Check sheet for the modelled part. Datum: model origin and axes. Units: mm. A direction names the side the tool comes from. Coordinates: 2 decimals unless noted, no trailing zeros. Write each loop counter-clockwise with the first axis right and the second up, starting at its lowest first coordinate (ties: lowest second). Pieces come first, ordered by that corner, then holes. Notation, with made-up numbers: (-29.5, 58) -> (7.5, 58) arc R31 ccw to (7.5, 93) -> close; hole circle Ø2 at (15, 62.5). An arc over 180 degrees is marked (long way). One line per item, written item: value. Start each with the question number.
1) Sectioned sample at B-B on z = 23.5. Enter the section's corners in (x, y).
2) Sectioned sample at C-C on x = -4. Enter the section's corners in (y, z).
3) Set-up check for faces 1 (the flat face through (-20, 0, 20)), 2 (the cylindrical face through (-53.987, 14.298, 5.07)), 3 (the flat face through (31, 5, 10)): record each of +Z, -Z, +X, -X, +Y, -Y from which the full face is reachable in a straight line by a thin tool's end or side.
4) Sectioned sample at A-A on y = 7. Give the number of separate pieces and of enclosed holes in the cut face, plus the area to 3 significant figures.
5) Scan lines: line 1 along X through (y, z) = (0, 4); line 2 along Y through (x, z) = (40, 4); line 3 along Z through (x, y) = (0, 4.5). Record each from-to range of solid material in increasing order. Write a range as [from, to].
6) Gauge pin test, flat ends, axial feed: P1, Ø2, axis at y = -16, z = 18, coming from the +X side; P2, Ø10, axis at y = -11, z = 33, coming from the -X side; P3, Ø18, axis at x = 40, y = 0, coming from the +Z side; P4, Ø5, axis at y = -6.5, z = 6, coming from the -X side. Record the tip position at first contact, or that the pin passes through.
7) Draft check along Y on faces 4 (the flat face through (-27, 0, 10)), 5 (the cylindrical face through (53.987, -14.298, 5.07)), 6 (the cylindrical face through (49.76, -2.17, 5.07)). Enter one of: +Y half, -Y half, draft (parallel to the pull), parting line (faces both ways), or undercut.
Autodesk Fusion 360 part; units mm, degrees
sketch "Sketch1" plane through (0, 0, 0) normal (0, 0, 1) x (1, 0, 0)
  line L0 (40, 20) -> (-40, 20)
  line L1 (-40, 20) -> (-40, -20)
  line L2 (-40, -20) -> (40, -20)
  line L3 (40, -20) -> (40, 20)
  line L4 (40, 20) -> (-40, -20) construction
  line L5 (-40, 20) -> (40, -20) construction
  line L6 (-40, -20) -> (-20, -20) construction
  line L7 (-40, -20) -> (-20, -20) construction
  line L8 (40, -20) -> (20, -20) construction
  line L9 (-20, -20) -> (-20, 20)
  line L10 (20, -20) -> (20, 20)
  line L11 (-40, -20) -> (-60, -20)
  line L12 (-40, 20) -> (-60, 20)
  line L13 (-60, 20) -> (-60, -20)
  line L14 (40, 20) -> (60, 20)
  line L15 (60, 20) -> (60, -20)
  line L16 (60, -20) -> (40, -20)
  line L17 (-40, 0) -> (-40, 20) construction
  line L18 (40, 20) -> (40, 0) construction
  dimension "d1" = 80
  dimension "d2" = 40
  dimension "d3" = 20
  dimension "d4" = 20
  dimension "d5" = 20
extrude "Extrude2" add sketch "Sketch1" along normal blind 50 contours L0 L2 L9 L10 makes body 1
extrude "Extrude1" add sketch "Sketch1" along normal blind 10 separate body contours L0 L2 L3 L10 | L3 L14 L15 L16 | L0 L1 L2 L9 | L1 L11 L12 L13 makes body 2 at (-33.3333, -6.6667, 0) makes body 3 at (46.6667, -6.6667, 0)
fillet "Fillet1" radius 20 4 edges at (-60, -20, 5) (-60, 20, 5) (60, -20, 5) (60, 20, 5) on bodies 2 3
hole "Hole1" at (-40, 0, 0) direction (0, 0, 1) diameter 20 depth 10 tip angle 118 bodies 2
hole "Hole2" at (40, 0, 0) direction (0, 0, 1) diameter 20 depth 10 tip angle 118 bodies 3
fillet "Fillet2" radius 20 2 edges at (-20, 0, 50) (20, 0, 50) on bodies 1
sketch "Sketch2" plane through (0, -20, 0) normal (0, -1, 0) x (1, 0, 0)
  arc A0 (20, 30) -> (-20, 30) centre (0, 30) ccw
  line L0 (-20, 30) -> (-20, 0)
  line L1 (-20, 0) -> (20, 0)
  line L2 (20, 0) -> (20, 30)
  line L3 (-20, 30) -> (20, 30) construction
hole "Hole3" at (0, -20, 30) direction (0, 1, 0) diameter 20 depth 40 tip angle 118 bodies 1
combine "Combine1" operation add target body 2 tool bodies 3 1
Answers:
1. outline: (-20, -20) -> (-7.6, -20) -> (-7.6, 20) -> (-20, 20) -> close; (7.6, -20) -> (20, -20) -> (20, 20) -> (7.6, 20) -> close
2. outline: (-20, 0) -> (20, 0) -> (20, 20.83) -> (-20, 20.83) -> close; (-20, 39.17) -> (20, 39.17) -> (20, 49.6) -> (-20, 49.6) -> close
3. face 1: +Z, -X, +Y, -Y
3. face 2: +Z, -Z, -X, +Y
3. face 3: +Z, +X, +Y, -Y
4. separate pieces: 3
4. enclosed holes: 1
4. area: 2,000 mm2
5. line 1: x = [-60, -50], [-30, 30], [50, 60]
5. line 2: y = [-20, -10], [10, 20]
5. line 3: z = [0, 20], [40, 50]
6. P1: stops at x = 20
6. P2: stops at x = -20
6. P3: passes through
6. P4: stops at x = -59.6
7. face 4: draft
7. face 5: -Y half
7. face 6: undercut
